from build123d import *

# Parameters (mm, degrees)
CROQUIS1_W            = 4
CROQUIS1_H            = 6
CHAFL_N1_SIZE         = 0.5
CORTAR_EXTRUIR1_DEPTH = 4


with BuildPart() as part:
    # Croquis1 → Revolución1 (revolve)
    with BuildSketch(Plane.XY, mode=Mode.PRIVATE) as revoluci_n1_sk:
        with Locations((2, -3)):
            Rectangle(CROQUIS1_W, CROQUIS1_H)
    revolve(revoluci_n1_sk.sketch.rotate(Axis((0, 0, 0), (0, -1, 0)), 90), axis=Axis((0, 0, 0), (0, -1, 0)))

    # Chaflán1
    chafl_n1_edges = [part.edges().sort_by_distance(p)[0] for p in [
        (0, -6, -4),
        (0, 0, -4),
    ]]
    chamfer(chafl_n1_edges, length=CHAFL_N1_SIZE)

    # Croquis2 → Cortar-Extruir1 (cut)
    with BuildSketch(Plane.XZ.offset(6)):
        Polygon((-1.154700538, -2), (1.154700538, -2), (2.309401077, 0), (1.154700538, 2), (-1.154700538, 2), (-2.309401077, 0), align=None)
    extrude(amount=-CORTAR_EXTRUIR1_DEPTH, mode=Mode.SUBTRACT)


solid = part.part
Read the model definition and answer for the solid it produces. Units are mm, in the model's axes. A direction names the side the tool comes from. Coordinates: 2 decimals unless noted, no trailing zeros. Loops run counter-clockwise (first coordinate to the right, second up) from the corner with the lowest first, then second, coordinate; pieces in that order, holes last. Notation, with made-up numbers: (12.25, 62) - (63.25, 62) arc R21 cw to (63.25, 89) - close; hole circle Ø5 at (-22.75, 41). An arc over 180 degrees is marked (long way). Answer in a Markdown table with one row per item.
Q1. Given P1, Ø3, axis at x = -0.5, z = 0, coming from the -Y side; P2, Ø1.5, axis at y = -4.5, z = -2, coming from the +X side; P3, Ø1, axis at x = 3, y = -1.5, coming from the -Z side, each flat-ended and moving along its own axis, determine where each tip first touches the part or whether it passes through.
Here are the results:
| item | result |
|---|---|
| P1 | stops at y = -2 |
| P2 | stops at x = 3.8 |
| P3 | stops at z = -3.12 |
Q2. For faces 5 (the flat face through (2, -6, -2)), 6 (the flat face through (1.74, -4.03, 0.99)), determine the directions among +Z, -Z, +X, -X, +Y, -Y from which every point of the face is accessible in a straight line to the end or side of a thin tool.
Here are the results:
| item | result |
|---|---|
| face 5 | +Z, -Z, +X, -X, -Y |
| face 6 | -Y |
Q3. Find section A-A on y = -4.75. Write down the section's boundary in (x, z).
Here are the results:
| item | result |
|---|---|
| outline | circle Ø8 at (0, 0); hole (-2.31, 0) - (-1.15, -2) - (1.15, -2) - (2.31, 0) - (1.15, 2) - (-1.15, 2) - close |
Q4. The mould has two halves that part along Z. Classify faces 1 (the cylindrical face through (3.905, -2.965, -0.867)), 2 (the flat face through (-1.74, -4.03, -0.99)), 3 (the flat face through (0, 0, 0)), 4 (the flat face through (0, -4, -2)): pulls with the +Z half, pulls with the -Z half, needs draft (parallel to the pull), parting line crosses it, or undercut.
Here are the results:
| item | result |
|---|---|
| face 1 | parting line crosses it |
| face 2 | undercut |
| face 3 | needs draft |
| face 4 | undercut |
Q5. Straight lines are drawn through the part: line 1 along Y through (x, z) = (0, 1.25); line 2 along Z through (x, y) = (-1.5, -2.3); line 3 along X through (y, z) = (-4.85, -1.75). For each, find the intervals that lie inside material, in ascending order. Write a range as [from, to].
Here are the results:
| item | result |
|---|---|
| line 1 | y = [-2, 0] |
| line 2 | z = [-3.71, -1.4], [1.4, 3.71] |
| line 3 | x = [-3.6, -1.3], [1.3, 3.6] |
